```python
from build123d import *

# Parameters (mm, degrees)
BASE_FLANGE1_DEPTH   = 17.5
M5_CLEARANCE_HOLE2_D = 5.8
M5_CLEARANCE_HOLE1_D = 5.8
CUT_EXTRUDE3_DEPTH   = 2
SKETCH21_R           = 1.75
BOSS_EXTRUDE1_DEPTH  = 2
SKETCH22_W           = 6
SKETCH22_H           = 52
CUT_EXTRUDE4_DEPTH   = 10
FILLET1_R            = 2
FILLET2_R            = 10


# Sheet-metal steps are written as plain solids
with BuildPart() as part:
    # Sketch1 → Base-Flange1 (new, symmetric)
    with BuildSketch(Plane.XY):
        with BuildLine():
            Line((0, 100), (0, 4))
            ThreePointArc((0, 4), (1.171572875, 1.171572875), (4, 0))
            Line((4, 0), (19, 0))
            Line((19, 0), (19, 2))
            Line((19, 2), (4, 2))
            ThreePointArc((4, 2), (2.585786438, 2.585786438), (2, 4))
            Line((2, 4), (2, 100))
            Line((2, 100), (0, 100))
        make_face()
    extrude(amount=BASE_FLANGE1_DEPTH, both=True)

    # M5 Clearance Hole2 (through all)
    with Locations(Plane(origin=(0, 2, 0), x_dir=(1, 0, 0), z_dir=(0, 1, 0))):
        with Locations((13, -12.5), (13, 12.5)):
            Hole(M5_CLEARANCE_HOLE2_D / 2)

    # M5 Clearance Hole1 (through all)
    with Locations(Plane(origin=(2, 0, 0), x_dir=(0, 0, -1), z_dir=(1, 0, 0))):
        with Locations((0, 92), (0, 42)):
            Hole(M5_CLEARANCE_HOLE1_D / 2)

    # Sketch20 → Cut-Extrude3 (cut)
    with BuildSketch(Plane(origin=(2, 0, 0), x_dir=(0, 0, -1), z_dir=(1, 0, 0))):
        Polygon((-10, 100), (-10, 19.990381057), (-17.5, 7), (-17.5, 100), align=None)
    cut_extrude3 = extrude(amount=-CUT_EXTRUDE3_DEPTH, mode=Mode.SUBTRACT)

    # Mirror1: Cut-Extrude3 across plane
    add(cut_extrude3.mirror(Plane.XY), mode=Mode.SUBTRACT)

    # Sketch21 → Boss-Extrude1 (add)
    with BuildSketch(Plane(origin=(0, 2, 0), x_dir=(1, 0, 0), z_dir=(0, 1, 0))):
        Polygon((4, -17.5), (19, -17.5), (19, 0), (25.6, 0), (25.6, -17.5), (25.6, -34), (4, -34), align=None)
        with Locations(Location((9.6, -30, 0), (0, 0, 270))):
            Circle(SKETCH21_R, mode=Mode.SUBTRACT)
        with Locations(Location((21.6, -30, 0), (0, 0, 270))):
            Circle(SKETCH21_R, mode=Mode.SUBTRACT)
    boss_extrude1 = extrude(amount=-BOSS_EXTRUDE1_DEPTH)

    # Mirror2: Boss-Extrude1 across plane
    add(boss_extrude1.mirror(Plane.XY))

    # Sketch22 → Cut-Extrude4 (cut)
    with BuildSketch(Plane(origin=(0, 2, 0), x_dir=(1, 0, 0), z_dir=(0, 1, 0))):
        with Locations((22.6, 0)):
            Rectangle(SKETCH22_W, SKETCH22_H)
    extrude(amount=-CUT_EXTRUDE4_DEPTH, mode=Mode.SUBTRACT)

    # Fillet1
    fillet1_edges = [part.edges().sort_by_distance(p)[0] for p in [
        (4, 1, 34),
        (25.6, 1, 34),
        (4, 1, -34),
        (25.6, 1, -34),
        (25.6, 1, -26),
        (25.6, 1, 26),
        (19.6, 1, 26),
        (19.6, 1, -26),
    ]]
    fillet(fillet1_edges, radius=FILLET1_R)

    # Fillet2
    fillet2_edges = [part.edges().sort_by_distance(p)[0] for p in [
        (1, 7, 17.5),
        (1, 7, -17.5),
        (1, 19.990381057, 10),
        (1, 19.990381057, -10),
        (1, 100, 10),
        (1, 100, -10),
    ]]
    fillet(fillet2_edges, radius=FILLET2_R - 0.0001)  # a hair under: the kernel refuses the full size


solid = part.part
```
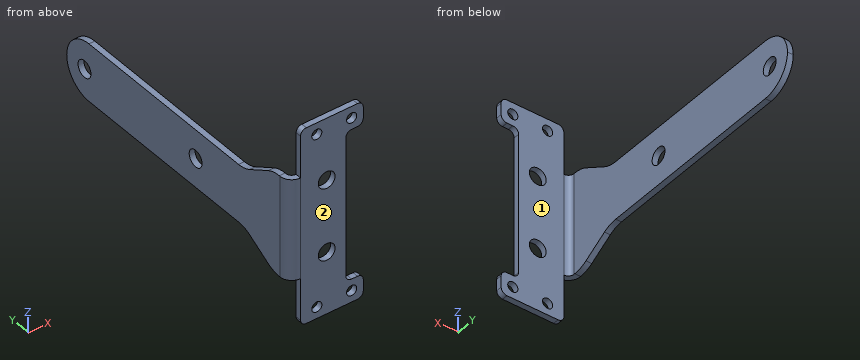
Geometry: final body of the model. Coordinates: model frame, mm. Face numbers are marked on the shaded views. A direction names the side the tool comes from. Give positions to 0.01 mm unless a question says otherwise; leave off trailing zeros. Write each loop counter-clockwise with the first axis right and the second up, starting at its lowest first coordinate (ties: lowest second). Pieces come first, ordered by that corner, then holes.
1. Section query D-D, the plane z = 13.5. Return loops of the section in (x, y), then the cut area to 3 significant figures.
2. Section query A-A, the plane y = 42. Return loops of the section in (x, z).
3. Reachability of the marked faces 1 and 2 from +Z, -Z, +X, -X, +Y, -Y: full face, straight path, thin tool, end or side. Return the list, or none.
4. Pin query (flat end, axial travel): P1, Ø2, axis at x = 9.6, z = -30, coming from the -Y side; P2, Ø5, axis at x = 8, z = 22, coming from the +Y side; P3, Ø3, axis at x = 1, y = 3, coming from the +Z side; P4, Ø17.5, axis at y = 74, z = -1, coming from the +X side. Return the tip coordinate at first contact, or that it passes through.
5. Section query C-C, the plane z = 30. Return loops of the section in (x, y).
6. Line query: probe 1 along X at (y, z) = (1.6, -30); probe 2 along Z at (x, y) = (13, 1.3); probe 3 along Y at (x, z) = (18.25, 16). Output: solid intervals per line, ascending.
7. Section query B-B, the plane x = 13. Return loops of the section in (y, z).
Computed:
1. outline: (0, 4) arc R4 ccw to (4, 0) - (10.28, 0) - (10.28, 2) - (4, 2) arc R2 cw to (2, 4) - (2, 13.93) - (0, 13.93) - close; (15.72, 0) - (19.6, 0) - (19.6, 2) - (15.72, 2) - close
1. area: 49.6 mm2
2. outline: (0, -10) - (2, -10) - (2, -2.9) - (0, -2.9) - close; (0, 2.9) - (2, 2.9) - (2, 10) - (0, 10) - close
3. face 1: +Z, -Z, +X, +Y
3. face 2: +Z, -Z, +X, -X, -Y
4. P1: passes through
4. P2: stops at y = 2
4. P3: stops at z = 17.5
4. P4: stops at x = 2
5. outline: (4, 0) - (7.85, 0) - (7.85, 2) - (4, 2) - close; (11.35, 0) - (19.85, 0) - (19.85, 2) - (11.35, 2) - close; (23.35, 0) - (25.6, 0) - (25.6, 2) - (23.35, 2) - close
6. probe 1: x = 4 to 7.85, 11.35 to 19.85, 23.35 to 25.6
6. probe 2: z = -34 to -15.4, -9.6 to 9.6, 15.4 to 34
6. probe 3: y = 0 to 2
7. outline: (0, -34) - (2, -34) - (2, -15.4) - (0, -15.4) - close; (0, -9.6) - (2, -9.6) - (2, 9.6) - (0, 9.6) - close; (0, 15.4) - (2, 15.4) - (2, 34) - (0, 34) - close
